The model under review builds one solid part; all positions refer to its coordinate system, in mm. A direction names the side the tool comes from. Give positions to 0.01 mm unless a question says otherwise; leave off trailing zeros. Write each loop counter-clockwise with the first axis right and the second up, starting at its lowest first coordinate (ties: lowest second). Pieces come first, ordered by that corner, then holes. Notation, with made-up numbers: (24, -17.5) -> (59, -17.5) arc R17 ccw to (59, 6.5) -> close; hole circle Ø9 at (81, 76). An arc over 180 degrees is marked (long way). Use CSV: the item, a comma, the result in double quotes.
```python
from build123d import *

# Parameters (mm, degrees)
F1_DEPTH = 95
F2_DEPTH = 10
F4_START = 10
F3_W     = 6.5
F3_H     = 5
F4_DEPTH = 2
F5_START = -10
F3_W_2   = 13
F5_DEPTH = 2


with BuildPart() as f1:
    # F0 (on Front) → F1 (new body)
    with BuildSketch(Plane.XZ):
        with BuildLine():
            Line((-10, -8), (10, -8))
            ThreePointArc((10, -8), (11.4142135624, -7.4142135624), (12, -6))
            Line((12, -6), (12, 6))
            ThreePointArc((12, 6), (11.4142135624, 7.4142135624), (10, 8))
            Line((10, 8), (-10, 8))
            ThreePointArc((-10, 8), (-11.4142135624, 7.4142135624), (-12, 6))
            Line((-12, 6), (-12, -6))
            ThreePointArc((-12, -6), (-11.4142135624, -7.4142135624), (-10, -8))
        make_face()
        Polygon((-2, 5), (-2, 6), (2, 6), (2, 5), (3.5, 5), (3.5, 3), (6, 3), (6, -4), (-6, -4), (-6, 3), (-3.5, 3), (-3.5, 5), align=None, mode=Mode.SUBTRACT)
        Polygon((2, 6), (-2, 6), (-2, 5), (-3.5, 5), (-3.5, 3), (-6, 3), (-6, -4), (6, -4), (6, 3), (3.5, 3), (3.5, 5), (2, 5), align=None)
    extrude(amount=-F1_DEPTH)

    # F0 (on Front) → F2 (cut)
    with BuildSketch(Plane.XZ):
        Polygon((2, 6), (-2, 6), (-2, 5), (-3.5, 5), (-3.5, 3), (-6, 3), (-6, -4), (6, -4), (6, 3), (3.5, 3), (3.5, 5), (2, 5), align=None)
    extrude(amount=-F2_DEPTH, mode=Mode.SUBTRACT)

    # F3 (on Right) → F4 (cut)
    with BuildSketch(Plane.YZ.offset(F4_START)):
        with Locations((85.75, 0.5)):
            Rectangle(F3_W, F3_H)
    extrude(amount=F4_DEPTH, mode=Mode.SUBTRACT)

    # F3 (on Right) → F5 (cut)
    with BuildSketch(Plane.YZ.offset(F5_START)):
        with Locations((74.5, -1.5)):
            Rectangle(F3_W_2, F3_H)
        with Locations((56, -1.5)):
            Rectangle(F3_W_2, F3_H)
        with Locations((37.5, -1.5)):
            Rectangle(F3_W_2, F3_H)
    extrude(amount=-F5_DEPTH, mode=Mode.SUBTRACT)


solid = f1.part
```
Q1. The part is to be moulded in two halves that separate along Y. For faces 5 (the flat face through (3.5, 5, 4)), 6 (the flat face through (-11, 44, -2)), say which applies: pulls with the +Y half, pulls with the -Y half, needs draft (parallel to the pull), parting line crosses it, or undercut.
Derived:
face 5,"needs draft"
face 6,"undercut"
Q2. Machinability: for faces 1 (the flat face through (0, 47, -8)), 2 (the flat face through (-6, 5, 0)), 3 (the flat face through (11, 86, -2)), 4 (the flat face through (-11, 81, -2)), which of the approach directions +Z, -Z, +X, -X, +Y, -Y give a long, thin tool a straight path to every point of the face, cutting with its end or side? Answer none if there is none.
Derived:
face 1,"-Z, +X, -X, +Y, -Y"
face 2,"-Y"
face 3,"+X"
face 4,"-X"
Q3. Insertion check: pin 1 (1.6 mm diameter, centred on x = 11, y = 86, fed in from -Z); pin 2 (1 mm diameter, centred on x = 1.5, z = 3.5, fed in from -Y); pin 3 (1.6 mm diameter, centred on x = 11, y = 87, fed in from +Z). Each pin has a flat end and moves straight along its axis. Give the tip position at first contact, or say it passes through.
Derived:
pin 1,"stops at z = -7.99"
pin 2,"stops at y = 10"
pin 3,"stops at z = 7.99"
Q4. To check wall thickness, follow probe 1 along Z at (x, y) = (2.5, 8.5); probe 2 along X at (y, z) = (31.5, -3.5); probe 3 along Y at (x, z) = (0, -2.5). State the ranges of each line that lie inside material, in increasing order.
Derived:
probe 1,"z = -8 to -4, 5 to 8"
probe 2,"x = -10 to 12"
probe 3,"y = 10 to 95"
Q5. Consider section C-C (y = 59). Write out the cut boundary in (x, z), then the cut area to 3 significant figures.
Derived:
outline,"(-12, -6) arc R2 ccw to (-10, -8) -> (10, -8) arc R2 ccw to (12, -6) -> (12, 6) arc R2 ccw to (10, 8) -> (-10, 8) arc R2 ccw to (-12, 6) -> (-12, 1) -> (-10, 1) -> (-10, -4) -> (-12, -4) -> close"
area,"371 mm2"
Q6. Consider section D-D (y = 9). Write out the cut boundary in (x, z), then the cut area to 3 significant figures.
Derived:
outline,"(-12, -6) arc R2 ccw to (-10, -8) -> (10, -8) arc R2 ccw to (12, -6) -> (12, 6) arc R2 ccw to (10, 8) -> (-10, 8) arc R2 ccw to (-12, 6) -> close; hole (-6, -4) -> (6, -4) -> (6, 3) -> (3.5, 3) -> (3.5, 5) -> (2, 5) -> (2, 6) -> (-2, 6) -> (-2, 5) -> (-3.5, 5) -> (-3.5, 3) -> (-6, 3) -> close"
area,"279 mm2"
Q7. Consider section B-B (x = 5). Write out the cut boundary in (y, z).
Derived:
outline,"(0, -8) -> (95, -8) -> (95, 8) -> (0, 8) -> (0, 3) -> (10, 3) -> (10, -4) -> (0, -4) -> close"
Q8. Consider section A-A (z = -0.25). Write out the cut boundary in (x, y).
Derived:
outline,"(-12, 0) -> (-6, 0) -> (-6, 10) -> (6, 10) -> (6, 0) -> (12, 0) -> (12, 82.5) -> (10, 82.5) -> (10, 89) -> (12, 89) -> (12, 95) -> (-12, 95) -> (-12, 81) -> (-10, 81) -> (-10, 68) -> (-12, 68) -> (-12, 62.5) -> (-10, 62.5) -> (-10, 49.5) -> (-12, 49.5) -> (-12, 44) -> (-10, 44) -> (-10, 31) -> (-12, 31) -> close"
